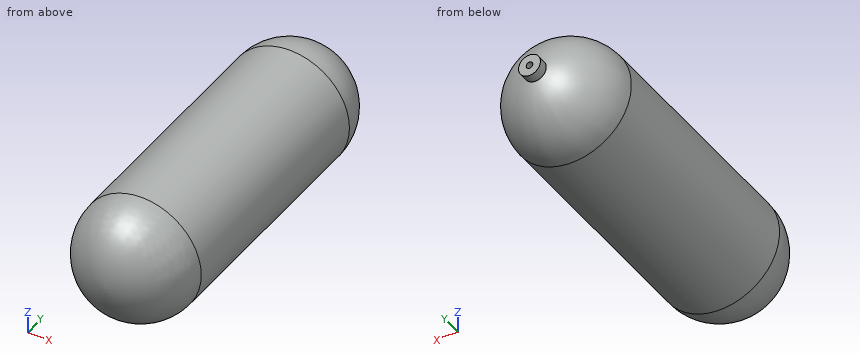
from build123d import *

# Parameters (mm, degrees)
SKETCH2_R                        = 15.875
BOSS_EXTRUDE1_DEPTH              = 12.7
BOSS_EXTRUDE1_DIRECTION_2_REACH  = 535.4
F_3_8_0_375_DIAMETER_HOLE1_D     = 9.525
F_3_8_0_375_DIAMETER_HOLE1_DEPTH = 25.4
F_3_8_0_375_DIAMETER_HOLE1_TIP   = 2.861599


with BuildPart() as part:
    # Sketch1 → Revolve1 (revolve)
    with BuildSketch(Plane.XY):
        with BuildLine():
            Line((87.63, 445.77), (87.63, 87.63))
            ThreePointArc((87.63, 87.63), (61.963767, 25.666233), (0, 0))
            Line((0, 0), (0, 3.175))
            ThreePointArc((0, 3.175), (59.718703, 27.911297), (84.455, 87.63))
            Line((84.455, 87.63), (84.455, 445.77))
            ThreePointArc((84.455, 445.77), (59.718703, 505.488703), (0, 530.225))
            Line((0, 530.225), (0, 533.4))
            ThreePointArc((0, 533.4), (61.963767, 507.733767), (87.63, 445.77))
        make_face()
    revolve(axis=Axis((0, 533.4, 0), (0, 1, 0)))

    # Sketch2 → Boss-Extrude1 (add)
    with BuildSketch(Plane(origin=(0, 533.4, 0), x_dir=(1, 0, 0), z_dir=(0, 1, 0))):
        Circle(SKETCH2_R)
    extrude(amount=BOSS_EXTRUDE1_DEPTH)

    # Sketch2 → Boss-Extrude1 direction 2 (add, up to next)
    with BuildSketch(Plane(origin=(0, 533.4, 0), x_dir=(1, 0, 0), z_dir=(0, 1, 0)), mode=Mode.PRIVATE) as boss_extrude1_direction_2_sk1:
        Circle(SKETCH2_R)
    boss_extrude1_direction_2_tool1 = extrude(boss_extrude1_direction_2_sk1.sketch, amount=-BOSS_EXTRUDE1_DIRECTION_2_REACH, mode=Mode.PRIVATE) - part.part
    add(boss_extrude1_direction_2_tool1.solids().sort_by_distance((0, 533.4, 0))[0])

    # 3/8 (0.375) Diameter Hole1
    with Locations(Plane(origin=(-0.053239, 546.1, 0.093777), x_dir=(0, 0, 1), z_dir=(0, 1, 0))):
        with Locations((0, 0)):
            Hole(F_3_8_0_375_DIAMETER_HOLE1_D / 2, depth=F_3_8_0_375_DIAMETER_HOLE1_DEPTH)
            with Locations((0, 0, -(F_3_8_0_375_DIAMETER_HOLE1_DEPTH + F_3_8_0_375_DIAMETER_HOLE1_TIP / 2))):  # 118° drill point
                Cone(0, F_3_8_0_375_DIAMETER_HOLE1_D / 2, F_3_8_0_375_DIAMETER_HOLE1_TIP, mode=Mode.SUBTRACT)


solid = part.part
Work out the finished part from the listing and answer in its coordinate system (mm). Give positions to 0.01 mm unless a question says otherwise; leave off trailing zeros. Loops run counter-clockwise (first coordinate to the right, second up) from the corner with the lowest first, then second, coordinate; pieces in that order, holes last. Notation, with made-up numbers: (-32, -16) - (7, -16) arc R19 ccw to (7, 1) - close; hole circle Ø5 at (-39, 2.5). An arc over 180 degrees is marked (long way). Answer in a Markdown table with one row per item.
(1) Consider L1, parallel to Z at x = 0, y = 314 (3 decimals); L2, parallel to Z at x = 4, y = 259. Determine where each line is inside the solid, lowest interval first. Write a range as [from, to].
Results list:
| item | result |
|---|---|
| L1 | z = [-87.63, -84.455], [84.455, 87.63] |
| L2 | z = [-87.54, -84.36], [84.36, 87.54] |
(2) Flat-ended cylindrical pins translate along their axes: pin 1 Ø1.5 at (x, y) = (-69, 302.5) entering from +Z; pin 2 Ø2 at (y, z) = (77.5, -26) entering from -X; pin 3 Ø2 at (x, y) = (19.5, 163) entering from -Z. Find the tip coordinate at first contact, or state that the pin passes through.
Results list:
| item | result |
|---|---|
| pin 1 | stops at z = 54.96 |
| pin 2 | stops at x = -83.4 |
| pin 3 | stops at z = -85.65 |
(3) Section A-A (y = 133) is taken. Give the vertices of the cut face in (x, z) (3 decimals), and give its area (3 significant figures).
Results list:
| item | result |
|---|---|
| outline | circle Ø175.26 at (0, 0); hole circle Ø168.91 at (0, 0) |
| area | 1,720 mm² |
